Design review of the part built by this model. Coordinates are the model's own, in mm. Face numbers are marked on the shaded views. Coordinates: 2 decimals unless noted, no trailing zeros. Loops run counter-clockwise (first coordinate to the right, second up) from the corner with the lowest first, then second, coordinate; pieces in that order, holes last. Notation, with made-up numbers: (5.25, 35.5) -> (43.25, 35.5) arc R4 ccw to (43.25, 40.5) -> close; hole circle Ø4 at (24.5, 48). An arc over 180 degrees is marked (long way). Answer as a JSON object with one key per item and string values.
```python
from build123d import *

# Parameters (mm, degrees)
F0_W     = 254
F0_H     = 762
F1_DEPTH = 152.4
F3_T     = -2.54
F4_W     = 248.92
F4_H     = 76.2
F5_DEPTH = 12.7


with BuildPart() as f1:
    # F0 (on Front) → F1 (new body)
    with BuildSketch(Plane.XZ):
        with Locations((-139.834513, 0.342414)):
            Rectangle(F0_W, F0_H)
    extrude(amount=F1_DEPTH)

    # F3
    f3_openings = [f1.faces().sort_by_distance(p)[0] for p in [
        (-139.834513, -76.2, 381.342414),
    ]]
    offset(amount=F3_T, openings=f3_openings)

    # F4 (on face) → F5 (cut)
    with BuildSketch(Plane.XZ.offset(152.4)):
        with Locations((-139.834513, -340.017586)):
            Rectangle(F4_W, F4_H)
    extrude(amount=-F5_DEPTH, mode=Mode.SUBTRACT)


solid = f1.part
```
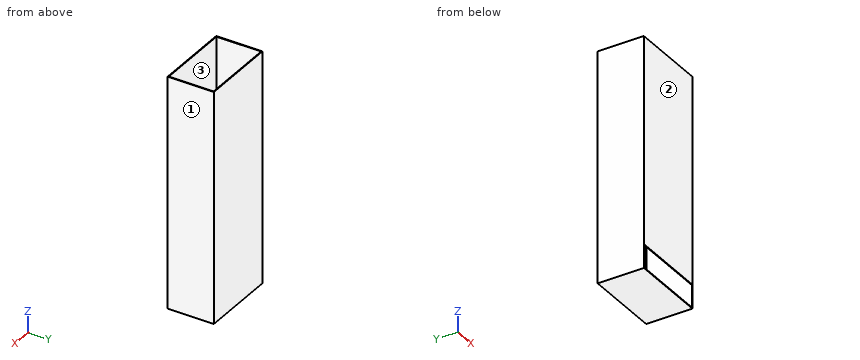
1) Add section A-A, the plane x = -125. Give the boundary of the cut face in (y, z), and give its area (3 significant figures).
Completed:
{"outline": "(-152.4, -380.66) -> (0, -380.66) -> (0, 381.34) -> (-2.54, 381.34) -> (-2.54, -378.12) -> (-152.4, -378.12) -> close; (-152.4, -301.92) -> (-149.86, -301.92) -> (-149.86, 381.34) -> (-152.4, 381.34) -> close", "area": "4,050 mm²"}
2) Add section D-D, the plane z = -335. Give the boundary of the cut face in (x, y), and give its area (3 significant figures).
Completed:
{"outline": "(-266.83, -152.4) -> (-264.29, -152.4) -> (-264.29, -2.54) -> (-15.37, -2.54) -> (-15.37, -152.4) -> (-12.83, -152.4) -> (-12.83, 0) -> (-266.83, 0) -> close", "area": "1,410 mm²"}
3) Clearance check with a flat-ended pin moving along its axis: pin 1 Ø3 at (x, y) = (-215, -53.5) entering from +Z. State where the tip first meets the part, or that it passes through.
Completed:
{"pin 1": "z = -378.12"}
4) Wall thickness on probe 1 along Y at (x, z) = (-54.5, -79); probe 2 along X at (y, z) = (-115.5, -318.5); probe 3 along Z at (x, y) = (-41, -117): over which ranges is each line inside the solid? List them lowest first.
Completed:
{"probe 1": "-152.4 to -149.86, -2.54 to 0", "probe 2": "-266.83 to -264.29, -15.37 to -12.83", "probe 3": "-380.66 to -378.12"}
5) The part is to be moulded in two halves that separate along X. For the marked faces 1, 2 and 3, say which applies: pulls with the +X half, pulls with the -X half, needs draft (parallel to the pull), parting line crosses it, or undercut.
Completed:
{"face 1": "pulls with the +X half", "face 2": "needs draft", "face 3": "undercut"}
6) Add section C-C, the plane y = -68.5. Give the boundary of the cut face in (x, z).
Completed:
{"outline": "(-266.83, -380.66) -> (-12.83, -380.66) -> (-12.83, 381.34) -> (-15.37, 381.34) -> (-15.37, -378.12) -> (-264.29, -378.12) -> (-264.29, 381.34) -> (-266.83, 381.34) -> close"}
7) Add section B-B, the plane z = -16.5. Give the boundary of the cut face in (x, y).
Completed:
{"outline": "(-266.83, -152.4) -> (-12.83, -152.4) -> (-12.83, 0) -> (-266.83, 0) -> close; hole (-264.29, -149.86) -> (-15.37, -149.86) -> (-15.37, -2.54) -> (-264.29, -2.54) -> close"}
